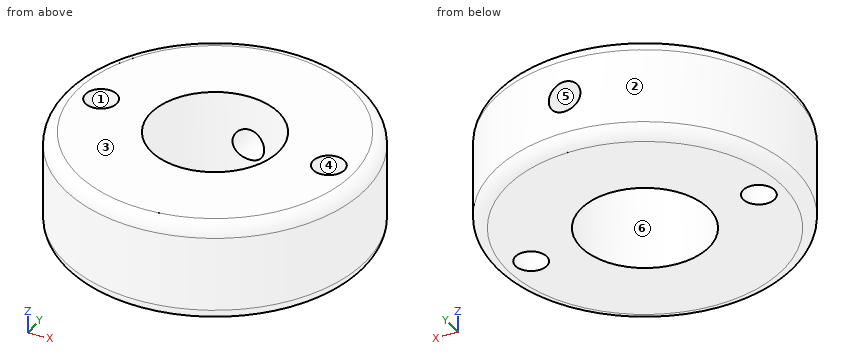
```python
from build123d import *

# Parameters (mm, degrees)
SKETCH1_W                    = 24
SKETCH1_H                    = 24
BOSS_EXTRUDE1_DEPTH          = 8
M3_TAPPED_HOLE1_D            = 2.5
F_10_2_10_2_DIAMETER_HOLE1_D = 10.2
M3_TAPPED_HOLE2_REACH        = 30
M3_TAPPED_HOLE2_BORE_R       = 1.25
SKETCH15_R                   = 18.5
SKETCH15_R_2                 = 12
CUT_EXTRUDE2_DEPTH           = 10
FILLET2_R                    = 1


with BuildPart() as part:
    # Sketch1 → Boss-Extrude1 (new body)
    with BuildSketch(Plane.XY):
        Rectangle(SKETCH1_W, SKETCH1_H)
    extrude(amount=BOSS_EXTRUDE1_DEPTH)

    # M3 Tapped Hole1 (through all)
    with Locations(Plane.XY.offset(8)):
        with Locations((9, 0), (-9, 0)):
            Hole(M3_TAPPED_HOLE1_D / 2)

    # Ø10.2 (10.2) Diameter Hole1 (through all)
    with Locations(Plane(origin=(0, 0, 0), x_dir=(-1, 0, 0), z_dir=(0, 0, -1))):
        with Locations((0, 0)):
            Hole(F_10_2_10_2_DIAMETER_HOLE1_D / 2)

    # M3 Tapped Hole2 bore → M3 Tapped Hole2 (cut, up to next)
    with BuildSketch(Plane(origin=(0, 12, 0), x_dir=(1, 0, 0), z_dir=(0, 1, 0)), mode=Mode.PRIVATE) as m3_tapped_hole2_sk1:
        with Locations((0, -4)):
            Circle(M3_TAPPED_HOLE2_BORE_R)
    m3_tapped_hole2_tool1 = extrude(m3_tapped_hole2_sk1.sketch, amount=-M3_TAPPED_HOLE2_REACH, mode=Mode.PRIVATE) & part.part
    add(m3_tapped_hole2_tool1.solids().sort_by_distance((0, 12, 4))[0], mode=Mode.SUBTRACT)

    # Sketch15 → Cut-Extrude2 (cut)
    with BuildSketch(Plane(origin=(0, 0, 0), x_dir=(-1, 0, 0), z_dir=(0, 0, -1))):
        Circle(SKETCH15_R)
        Circle(SKETCH15_R_2, mode=Mode.SUBTRACT)
    extrude(amount=-CUT_EXTRUDE2_DEPTH, mode=Mode.SUBTRACT)

    # Fillet2
    fillet2_edges = [part.edges().sort_by_distance(p)[0] for p in [
        (12, 0, 0),
        (12, 0, 8),
    ]]
    fillet(fillet2_edges, radius=FILLET2_R)


solid = part.part
```
Check sheet for the modelled part. Datum: model origin and axes. Units: mm. Face numbers are marked on the shaded views. A direction names the side the tool comes from. Coordinates: 2 decimals unless noted, no trailing zeros. Loops run counter-clockwise (first coordinate to the right, second up) from the corner with the lowest first, then second, coordinate; pieces in that order, holes last. Notation, with made-up numbers: M 71.25,89 L 126.25,89 A31 cw 126.25,128 Z; hole C 45,-13 d9. An arc over 180 degrees is marked long. Answer as a JSON object with one key per item and string values.
1. Sectioned sample at A-A on x = 0. Record the cut outline in (y, z).
Outcome:
{"outline": "M -12,1 A1 ccw -11,0 L -5.1,0 L -5.1,8 L -11,8 A1 ccw -12,7 Z; M 5.1,0 L 11,0 A1 ccw 12,1 L 12,2.75 L 5.1,2.75 Z; M 5.1,5.25 L 12,5.25 L 12,7 A1 ccw 11,8 L 5.1,8 Z"}
2. Sectioned sample at C-C on z = 4.5. Record the cut outline in (x, y).
Outcome:
{"outline": "M -1.15,4.97 L -1.15,11.95 A12 ccw long 1.15,11.95 L 1.15,4.97 A5.1 cw long Z; hole C -9,0 d2.5; hole C 9,0 d2.5"}
3. Sectioned sample at D-D on z = 2.25. Record the cut outline in (x, y), and give its area (3 significant figures).
Outcome:
{"outline": "C 0,0 d24; hole C -9,0 d2.5; hole C 0,0 d10.2; hole C 9,0 d2.5", "area": "361 mm²"}
4. Access from +Z, -Z, +X, -X, +Y, -Y to the whole of each face (thin tool, end or side, straight path). Record for the marked faces 5 and 6.
Outcome:
{"face 5": "+Y", "face 6": "+Z, -Z"}
5. Scan lines: L1, parallel to Z at x = 0, y = 6.75; L2, parallel to Y at x = 0, z = 6.5; L3, parallel to X at y = 9, z = 4. Record each from-to range of solid material in increasing order. Write a range as from..to.
Outcome:
{"L1": "0..2.75, 5.25..8", "L2": "-12..-5.1, 5.1..12", "L3": "-7.94..-1.25, 1.25..7.94"}
6. Release check for a two-part mould opening along X. For the marked faces 1, 2, 3 and 4 record: pulls with the +X half, pulls with the -X half, needs draft (parallel to the pull), parting line crosses it, or undercut.
Outcome:
{"face 1": "undercut", "face 2": "parting line crosses it", "face 3": "needs draft", "face 4": "undercut"}
7. Sectioned sample at B-B on y = 0. Record the cut outline in (x, z).
Outcome:
{"outline": "M -12,1 A1 ccw -11,0 L -10.25,0 L -10.25,8 L -11,8 A1 ccw -12,7 Z; M -7.75,0 L -5.1,0 L -5.1,8 L -7.75,8 Z; M 5.1,0 L 7.75,0 L 7.75,8 L 5.1,8 Z; M 10.25,0 L 11,0 A1 ccw 12,1 L 12,7 A1 ccw 11,8 L 10.25,8 Z"}
